Geometry: final body of the model. Coordinates: model frame, mm. Give positions to 0.01 mm unless a question says otherwise; leave off trailing zeros. Order: outer loops, then holes, each group sorted by start corner. A loop starts at its lowest first (then second) coordinate and runs counter-clockwise, first axis right, second up. Notation, with made-up numbers: M 22,-33.5 L 67,-33.5 A31 cw 67,-2.5 Z; hole C -33,5.5 d1. An arc over 180 degrees is marked long. Write item = value, one per line. Start each with the question number.
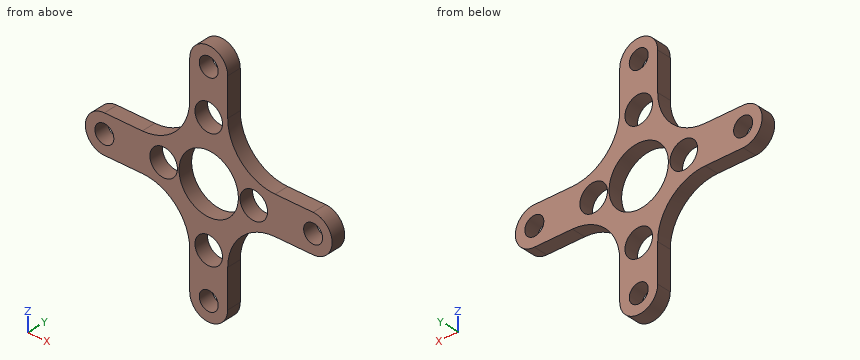
from build123d import *

# Parameters (mm, degrees)
IZIM2_R                     = 2
IZIM2_R_2                   = 2.9
IZIM2_R_3                   = 6.25
Y_KSEKLIK_EKSTR_ZYON1_DEPTH = 3


with BuildPart() as part:
    # Çizim2 → Yükseklik-Ekstrüzyon1 (new body)
    with BuildSketch(Plane(origin=(0, 0, 0), x_dir=(1, 0, 0), z_dir=(0, 1, 0))):
        with BuildLine():
            ThreePointArc((4, 22), (0, 26), (-4, 22))
            Line((-4, 22), (-4, 14))
            ThreePointArc((-4, 14), (-6.928932188, 6.928932188), (-14, 4))
            Line((-14, 4), (-22, 4))
            ThreePointArc((-22, 4), (-26, 0), (-22, -4))
            Line((-22, -4), (-14, -4))
            ThreePointArc((-14, -4), (-6.928932188, -6.928932188), (-4, -14))
            Line((-4, -14), (-4, -22))
            ThreePointArc((-4, -22), (0, -26), (4, -22))
            Line((4, -22), (4, -14))
            ThreePointArc((4, -14), (6.928932188, -6.928932188), (14, -4))
            Line((14, -4), (22, -4))
            ThreePointArc((22, -4), (26, 0), (22, 4))
            Line((22, 4), (14, 4))
            ThreePointArc((14, 4), (6.928932188, 6.928932188), (4, 14))
            Line((4, 14), (4, 22))
        make_face()
        with Locations(Location((0, -22, 0), (0, 0, 270))):
            Circle(IZIM2_R, mode=Mode.SUBTRACT)
        with Locations(Location((0, -12.5, 0), (0, 0, 270))):
            Circle(IZIM2_R_2, mode=Mode.SUBTRACT)
        with Locations(Location((-22, 0, 0), (0, 0, 270))):
            Circle(IZIM2_R, mode=Mode.SUBTRACT)
        with Locations(Location((-9.5, 0, 0), (0, 0, 270))):
            Circle(IZIM2_R_2, mode=Mode.SUBTRACT)
        with Locations(Location((0, 0, 0), (0, 0, 270))):
            Circle(IZIM2_R_3, mode=Mode.SUBTRACT)
        with Locations(Location((9.5, 0, 0), (0, 0, 270))):
            Circle(IZIM2_R_2, mode=Mode.SUBTRACT)
        with Locations(Location((0, 12.5, 0), (0, 0, 270))):
            Circle(IZIM2_R_2, mode=Mode.SUBTRACT)
        with Locations(Location((0, 22, 0), (0, 0, 270))):
            Circle(IZIM2_R, mode=Mode.SUBTRACT)
        with Locations(Location((22, 0, 0), (0, 0, 270))):
            Circle(IZIM2_R, mode=Mode.SUBTRACT)
    extrude(amount=Y_KSEKLIK_EKSTR_ZYON1_DEPTH)


solid = part.part
1) Ray query, L1, parallel to X at y = 0.8, z = 0; L2, parallel to X at y = 1.7, z = 22; L3, parallel to Z at x = -14, y = 0.5. Return the intervals inside material, ascending.
2) Cut plane C-C (x = -9.5). Return loops of the section in (y, z).
3) Cut plane D-D (x = 18.5). Return loops of the section in (y, z).
4) Cut plane B-B (y = 1.4). Give the number of separate pieces and of enclosed holes in the cut face, plus the area to 3 significant figures.
5) Pin query (flat end, axial travel): pin 1 Ø7.5 at (x, z) = (0, -12.5) entering from -Y; pin 2 Ø1.5 at (x, y) = (-20, 1.5) entering from +Z; pin 3 Ø1 at (y, z) = (1.5, 15) entering from -X; pin 4 Ø1.5 at (y, z) = (1.5, 18.5) entering from +X. Return the tip coordinate at first contact, or that it passes through.
6) Cut plane A-A (z = 12.5). Return loops of the section in (x, y).
Reply:
q1.L1 = -26 to -24, -20 to -12.4, -6.6 to -6.25, 6.25 to 6.6, 12.4 to 20, 24 to 26
q1.L2 = -4 to -2, 2 to 4
q1.L3 = -4 to 4
q2.outline = M 0,-5.07 L 3,-5.07 L 3,-2.9 L 0,-2.9 Z; M 0,2.9 L 3,2.9 L 3,5.07 L 0,5.07 Z
q3.outline = M 0,-4 L 3,-4 L 3,4 L 0,4 Z
q4.separate_pieces = 1
q4.enclosed_holes = 9
q4.area = 548 mm²
q5.pin_1 = 0
q5.pin_2 = 4
q5.pin_3 = -4
q5.pin_4 = 4
q6.outline = M -4.11,0 L -2.9,0 L -2.9,3 L -4.11,3 Z; M 2.9,0 L 4.11,0 L 4.11,3 L 2.9,3 Z
